from build123d import *

# Parameters (mm, degrees)
SKETCH1_W           = 119.38
SKETCH1_H           = 119.38
BOSS_EXTRUDE1_DEPTH = 25.4
CUT_EXTRUDE1_REACH  = 27.4
SKETCH2_R           = 2.165
FILLET1_R           = 7.5
FILLET2_R           = 7.5
FILLET3_R           = 7.5


with BuildPart() as part:
    # Sketch1 → Boss-Extrude1 (new body)
    with BuildSketch(Plane(origin=(0, 0, 0), x_dir=(1, 0, 0), z_dir=(0, 1, 0))):
        Rectangle(SKETCH1_W, SKETCH1_H)
    extrude(amount=BOSS_EXTRUDE1_DEPTH)

    # Sketch2 → Cut-Extrude1 (cut, up to next)
    with BuildSketch(Plane(origin=(0, 25.4, 0), x_dir=(1, 0, 0), z_dir=(0, 1, 0)), mode=Mode.PRIVATE) as cut_extrude1_sk1:
        with Locations((-52.19, 52.19)):
            Circle(SKETCH2_R)
    cut_extrude1_tool1 = extrude(cut_extrude1_sk1.sketch, amount=-CUT_EXTRUDE1_REACH, mode=Mode.PRIVATE) & part.part
    add(cut_extrude1_tool1.solids().sort_by_distance((-52.19, 25.4, -52.19))[0], mode=Mode.SUBTRACT)
    # Sketch2 → Cut-Extrude1 (cut, up to next)
    with BuildSketch(Plane(origin=(0, 25.4, 0), x_dir=(1, 0, 0), z_dir=(0, 1, 0)), mode=Mode.PRIVATE) as cut_extrude1_sk2:
        with Locations((52.19, 52.19)):
            Circle(SKETCH2_R)
    cut_extrude1_tool2 = extrude(cut_extrude1_sk2.sketch, amount=-CUT_EXTRUDE1_REACH, mode=Mode.PRIVATE) & part.part
    add(cut_extrude1_tool2.solids().sort_by_distance((52.19, 25.4, -52.19))[0], mode=Mode.SUBTRACT)
    # Sketch2 → Cut-Extrude1 (cut, up to next)
    with BuildSketch(Plane(origin=(0, 25.4, 0), x_dir=(1, 0, 0), z_dir=(0, 1, 0)), mode=Mode.PRIVATE) as cut_extrude1_sk3:
        with Locations((52.19, -52.19)):
            Circle(SKETCH2_R)
    cut_extrude1_tool3 = extrude(cut_extrude1_sk3.sketch, amount=-CUT_EXTRUDE1_REACH, mode=Mode.PRIVATE) & part.part
    add(cut_extrude1_tool3.solids().sort_by_distance((52.19, 25.4, 52.19))[0], mode=Mode.SUBTRACT)
    # Sketch2 → Cut-Extrude1 (cut, up to next)
    with BuildSketch(Plane(origin=(0, 25.4, 0), x_dir=(1, 0, 0), z_dir=(0, 1, 0)), mode=Mode.PRIVATE) as cut_extrude1_sk4:
        with Locations((-52.19, -52.19)):
            Circle(SKETCH2_R)
    cut_extrude1_tool4 = extrude(cut_extrude1_sk4.sketch, amount=-CUT_EXTRUDE1_REACH, mode=Mode.PRIVATE) & part.part
    add(cut_extrude1_tool4.solids().sort_by_distance((-52.19, 25.4, 52.19))[0], mode=Mode.SUBTRACT)

    # Fillet1
    fillet1_edges = [part.edges().sort_by_distance(p)[0] for p in [
        (-59.69, 12.7, -59.69),
    ]]
    fillet(fillet1_edges, radius=FILLET1_R)

    # Fillet2
    fillet2_edges = [part.edges().sort_by_distance(p)[0] for p in [
        (59.69, 12.7, -59.69),
    ]]
    fillet(fillet2_edges, radius=FILLET2_R)

    # Fillet3
    fillet3_edges = [part.edges().sort_by_distance(p)[0] for p in [
        (59.69, 12.7, 59.69),
        (-59.69, 12.7, 59.69),
    ]]
    fillet(fillet3_edges, radius=FILLET3_R)


solid = part.part
Read the model definition and answer for the solid it produces. Units are mm, in the model's axes. Give positions to 0.01 mm unless a question says otherwise; leave off trailing zeros. Answer as CSV lines item,"result". Start each with the question number.
1) This flat-tipped pin is pushed along its axis until it touches: pin 1 Ø4 at (x, z) = (52.19, 52.19) entering from -Y. Where does it stop, or does it pass through?
2) Determine the mould class of faces 1 (the face through (-1, 25.4, -1)), 2 (the face through (57.551, 12.878, 57.435)), 3 (the face through (53.19, 12.88, -50.27)) for opening direction X: released by +X, released by -X, zero draft, split by the parting line, or undercut.
3) Straight lines are drawn through the part: L1, parallel to X at y = 12, z = 52.19 (3 decimals); L2, parallel to Z at x = 51, y = 5.75. For each, find the intervals that lie inside material, in ascending order. Write a range as from..to.
Findings below:
1,pin 1,"through"
2,face 1,"zero draft"
2,face 2,"released by +X"
2,face 3,"undercut"
3,L1,"-59.69..-54.355, -50.025..50.025, 54.355..59.69"
3,L2,"-59.69..-54, -50.38..50.38, 54..59.69"
